Check sheet for the drawn part. Datum: minimum x, y, z corner. Units: mm. Give positions to 0.01 mm unless a question says otherwise; leave off trailing zeros. Loops run counter-clockwise (first coordinate to the right, second up) from the corner with the lowest first, then second, coordinate; pieces in that order, holes last. Notation, with made-up numbers: (10, 19) - (31, 19) arc R25 cw to (31, 41) - close; hole circle Ø3 at (26, 15.5). An arc over 180 degrees is marked (long way). Use a Markdown table: item, result. Add a question column.
1. Cross-section at D-D on y = 1.75. Enter the section's corners in (x, z), and give its area (3 significant figures).
2. Cross-section at C-C on z = 2.3. Enter the section's corners in (x, y), and give its area (3 significant figures).
3. Material ranges on L1, parallel to Z at x = 2.25, y = 3.75; L2, parallel to X at y = 3, z = 2.5; L3, parallel to Y at x = 21.5, z = 2.2, recorded low to high.
4. Depth check by flat-ended pin: P1, Ø0.8, axis at y = 5.5, z = 2.5, coming from the +X side; P2, Ø1.6, axis at x = 15, z = 2.5, coming from the +Y side; P3, Ø0.8, axis at x = 13.5, z = 2.5, coming from the -Y side. Enter the tip coordinate at first touch or a pass-through.
5. Cross-section at A-A on x = 11.25. Enter the section's corners in (y, z).
6. Cross-section at B-B on y = 4.25. Enter the section's corners in (x, z), and give its area (4 significant figures).
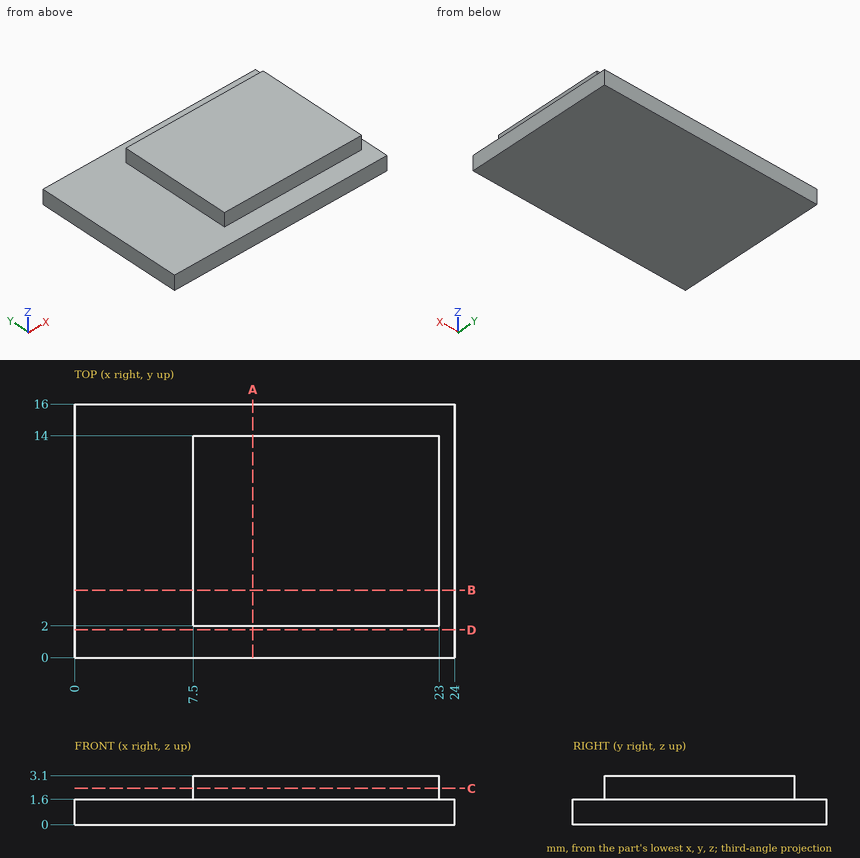
Values found:
| question | item | result |
|---|---|---|
| 1 | outline | (0, 0) - (24, 0) - (24, 1.6) - (0, 1.6) - close |
| 1 | area | 38.4 mm2 |
| 2 | outline | (7.5, 2) - (23, 2) - (23, 14) - (7.5, 14) - close |
| 2 | area | 186 mm2 |
| 3 | L1 | z = 0 to 1.6 |
| 3 | L2 | x = 7.5 to 23 |
| 3 | L3 | y = 2 to 14 |
| 4 | P1 | stops at x = 23 |
| 4 | P2 | stops at y = 14 |
| 4 | P3 | stops at y = 2 |
| 5 | outline | (0, 0) - (16, 0) - (16, 1.6) - (14, 1.6) - (14, 3.1) - (2, 3.1) - (2, 1.6) - (0, 1.6) - close |
| 6 | outline | (0, 0) - (24, 0) - (24, 1.6) - (23, 1.6) - (23, 3.1) - (7.5, 3.1) - (7.5, 1.6) - (0, 1.6) - close |
| 6 | area | 61.65 mm2 |
